from build123d import *

# Parameters (mm, degrees)
SKETCH1_W           = 50
SKETCH1_H           = 100
BOSS_EXTRUDE1_DEPTH = 2
SKETCH2_R           = 7
BOSS_EXTRUDE2_DEPTH = 100
SKETCH3_R           = 5
CUT_EXTRUDE1_DEPTH  = 114.624453084
FILLET3_R           = 7
SKETCH6_W           = 50
SKETCH6_H           = 10
CUT_EXTRUDE3_DEPTH  = 114.395398225
LPATTERN1_COUNT     = 5
LPATTERN1_PITCH     = 20
SKETCH7_R           = 1.75
CUT_EXTRUDE4_DEPTH  = 114.395398225
CHAMFER2_SIZE       = 1
LPATTERN3_COUNT     = 5
LPATTERN3_PITCH     = 20
CHAMFER3_SIZE       = 1


with BuildPart() as part:
    # Sketch1 → Boss-Extrude1 (new body)
    with BuildSketch(Plane(origin=(0, 0, 0), x_dir=(1, 0, 0), z_dir=(0, 1, 0))):
        with Locations((-25, 50)):
            Rectangle(SKETCH1_W, SKETCH1_H)
    extrude(amount=BOSS_EXTRUDE1_DEPTH)

    # Sketch2 → Boss-Extrude2 (add)
    with BuildSketch(Plane(origin=(0, 0, -100), x_dir=(-1, 0, 0), z_dir=(0, 0, -1))):
        with Locations((45.101020514, 7)):
            Circle(SKETCH2_R)
    extrude(amount=-BOSS_EXTRUDE2_DEPTH)

    # Sketch3 → Cut-Extrude1 (cut, through all)
    with BuildSketch(Plane(origin=(0, 0, -100), x_dir=(-1, 0, 0), z_dir=(0, 0, -1))):
        with Locations((45.101020514, 7)):
            Circle(SKETCH3_R)
    extrude(amount=-CUT_EXTRUDE1_DEPTH, mode=Mode.SUBTRACT)

    # Fillet3
    # the kernel refuses this fillet: 7 mm, written as the material it takes off along each edge
    with BuildSketch(Plane(origin=(-50, 0, 12.247448714), x_dir=(1, 0, 0), z_dir=(0, 0, -1))) as fillet3_piece_1:
        with BuildLine():
            CenterArc((4.898979486, -7), FILLET3_R, 90, 44.415308597)
            Line((0, -2), (-0.09797959, -1.9))
            ThreePointArc((-0.09797959, -1.9), (-0.14, -1), (-0.14, 0))
            Line((-0.14, 0), (0, 0.14))
            Line((0, 0.14), (4.898979486, 0.14))
            Line((4.898979486, 0.14), (4.898979486, 0))
        make_face()
    extrude(amount=124.494897428, mode=Mode.SUBTRACT)

    # Sketch6 → Cut-Extrude3 (cut, symmetric)
    with BuildSketch(Plane(origin=(0, 2, 0), x_dir=(1, 0, 0), z_dir=(0, 1, 0))):
        with Locations((-63.101020514, 85)):
            Rectangle(SKETCH6_W, SKETCH6_H)
    cut_extrude3 = extrude(amount=CUT_EXTRUDE3_DEPTH, both=True, mode=Mode.SUBTRACT)

    # LPattern1: Cut-Extrude3 ×5
    with Locations(*[(0, 0, i * LPATTERN1_PITCH) for i in range(1, LPATTERN1_COUNT)]):
        add(cut_extrude3, mode=Mode.SUBTRACT)

    # Sketch7 → Cut-Extrude4 (cut, symmetric)
    with BuildSketch(Plane(origin=(0, 2, 0), x_dir=(1, 0, 0), z_dir=(0, 1, 0))):
        with Locations(Location((-10, 90, 0), (0, 0, 270))):
            Circle(SKETCH7_R)
    cut_extrude4 = extrude(amount=CUT_EXTRUDE4_DEPTH, both=True, mode=Mode.SUBTRACT)

    # Chamfer2
    chamfer2_edges = [part.edges().sort_by_distance(p)[0] for p in [
        (-10, 2, -91.75),
    ]]
    chamfer(chamfer2_edges, length=CHAMFER2_SIZE)

    # LPattern3: Cut-Extrude4 ×5
    with Locations(*[(0, 0, i * LPATTERN3_PITCH) for i in range(1, LPATTERN3_COUNT)]):
        add(cut_extrude4, mode=Mode.SUBTRACT)

    # Chamfer3
    chamfer3_edges = [part.edges().sort_by_distance(p)[0] for p in [
        (-10, 2, -71.75),
        (-10, 2, -51.75),
        (-10, 2, -31.75),
        (-10, 2, -11.75),
    ]]
    chamfer(chamfer3_edges, length=CHAMFER3_SIZE)


solid = part.part
For this review, take the finished solid that the model builds, in its own axes (mm). A direction names the side the tool comes from. Round coordinates to 2 decimals unless told otherwise and drop trailing zeros. Write each loop counter-clockwise with the first axis right and the second up, starting at its lowest first coordinate (ties: lowest second). Pieces come first, ordered by that corner, then holes. Notation, with made-up numbers: (-35, -10) - (-6, -10) arc R17 ccw to (-6, -6) - close; hole circle Ø2 at (76, 67). An arc over 180 degrees is marked (long way). Use a Markdown table: item, result.
Q1. The part is to be moulded in two halves that separate along X. For faces 1 (the flat face through (-42, 2, -20)), 2 (the flat face through (-38.101, 1, -5)), 3 (the cylindrical face through (-9.474, 0.507, -8.331)), say which applies: pulls with the +X half, pulls with the -X half, needs draft (parallel to the pull), parting line crosses it, or undercut.
Derived:
| item | result |
|---|---|
| face 1 | needs draft |
| face 2 | pulls with the -X half |
| face 3 | undercut |
Q2. We need section C-C (z = -84.5). Give the boundary of the cut face in (x, y).
Derived:
| item | result |
|---|---|
| outline | (-38.1, 0) - (0, 0) - (0, 2) - (-38.1, 2) - close |
Q3. Clearance check with flat-ended pins moving along their axes: pin 1 (1 mm diameter, centred on y = 5.5, z = -30, fed in from -X); pin 2 (10 mm diameter, centred on x = -17, z = -79, fed in from +Y); pin 3 (1.6 mm diameter, centred on y = 0.5, z = -25.5, fed in from -X); pin 4 (2 mm diameter, centred on x = -10, z = -70, fed in from -Y) (3 decimals). State where each tip first meets the part, or that it passes through.
Derived:
| item | result |
|---|---|
| pin 1 | stops at x = -52.03 |
| pin 2 | stops at y = 2 |
| pin 3 | stops at x = -38.1 |
| pin 4 | passes through |
Q4. Wall thickness on line 1 along X through (y, z) = (6.75, -75.5); line 2 along Y through (x, z) = (-24, -4.5); line 3 along X through (y, z) = (8, -32): over which ranges is each line inside the solid? List them lowest first.
Derived:
| item | result |
|---|---|
| line 1 | x = -52.1 to -50.09, -40.11 to -38.11 |
| line 2 | y = 0 to 2 |
| line 3 | x = -52.03 to -50, -40.2 to -38.17 |
Q5. We need section A-A (x = -10). State how many separate pieces and enclosed holes the cut face has, plus the area to 3 significant figures.
Derived:
| item | result |
|---|---|
| separate pieces | 6 |
| enclosed holes | 0 |
| area | 160 mm2 |
Q6. We need section D-D (x = -3). Give the boundary of the cut face in (y, z), plus the area to 3 significant figures.
Derived:
| item | result |
|---|---|
| outline | (0, -100) - (2, -100) - (2, 0) - (0, 0) - close |
| area | 200 mm2 |
Q7. Machinability: for faces 4 (the flat face through (-42, 2, -90)), 5 (the cylindrical face through (-9.92, 0.51, -31.75)), 6 (the flat face through (-42, 2, -10)), which of the approach directions +Z, -Z, +X, -X, +Y, -Y give a long, thin tool a straight path to every point of the face, cutting with its end or side? Answer none if there is none.
Derived:
| item | result |
|---|---|
| face 4 | -X, +Y, -Y |
| face 5 | +Y, -Y |
| face 6 | +Z, -X, +Y, -Y |
